Part model, mm, in its own coordinate system. A direction names the side the tool comes from. Give positions to 0.01 mm unless a question says otherwise; leave off trailing zeros. Write each loop counter-clockwise with the first axis right and the second up, starting at its lowest first coordinate (ties: lowest second). Pieces come first, ordered by that corner, then holes.
```python
from build123d import *

# Parameters (mm, degrees)
F0_W     = 5
F0_H     = 200
F1_DEPTH = 300
F2_W     = 11
F2_H     = 7
F3_DEPTH = 300
F4_R     = 3.49999
F5_W     = 15
F5_H     = 31
F6_DEPTH = 7.001
F7_R     = 2
F8_W     = 8
F8_H     = 2
F9_DEPTH = 27
F10_R    = 1.99999


# Not quite as in the source:
# - a fillet or chamfer is up to 0.001 mm smaller than in the source, because OpenCascade refuses the exact size


with BuildPart() as f1:
    # F0 (on Front) → F1 (new body)
    with BuildSketch(Plane.XZ):
        with Locations((2.5, 100)):
            Rectangle(F0_W, F0_H)
    extrude(amount=F1_DEPTH)

    # F2 (on face) → F3 (join)
    with BuildSketch(Plane.XZ.offset(300)):
        with Locations((10.5, 3.5)):
            Rectangle(F2_W, F2_H)
    extrude(amount=-F3_DEPTH)

    # F4 (radius 3.5 in the source; OpenCascade refuses exactly that, so slightly less here)
    f4_edges = [f1.edges().sort_by_distance(p)[0] for p in [
        (16, -150, 7),
        (16, -150, 0),
    ]]
    fillet(f4_edges, radius=F4_R)

    # F5 (on face) → F6 (cut, through all)
    with BuildSketch(Plane.XY.offset(7)):
        with Locations((12.5, -284.5)):
            Rectangle(F5_W, F5_H)
        with Locations((12.5, -15.5)):
            Rectangle(F5_W, F5_H)
    extrude(amount=-F6_DEPTH, mode=Mode.SUBTRACT)

    # F7
    f7_edges = [f1.edges().sort_by_distance(p)[0] for p in [
        (2.5, -300, 200),
        (2.5, 0, 200),
        (2.5, -300, 0),
        (2.5, 0, 0),
    ]]
    fillet(f7_edges, radius=F7_R)

    # F8 (on face) → F9 (cut)
    with BuildSketch(Plane.XZ.offset(269)):
        with Locations((10.5, 4.5)):
            Rectangle(F8_W, F8_H)
    extrude(amount=-F9_DEPTH, mode=Mode.SUBTRACT)

    # F10 (radius 2 in the source; OpenCascade refuses exactly that, so slightly less here)
    f10_edges = [f1.edges().sort_by_distance(p)[0] for p in [
        (14.5, -255.5, 5.5),
    ]]
    fillet(f10_edges, radius=F10_R)


solid = f1.part
```
1) Saw through at B-B, the plane z = 117.5. Write the cut outline in (x, y), then the cut area to 3 significant figures.
Answers follow:
outline: (0, -300) - (5, -300) - (5, 0) - (0, 0) - close
area: 1,500 mm2
2) Wall check: L1, parallel to X at y = -170.5, z = 145; L2, parallel to Z at x = 8.5, y = -235; L3, parallel to Z at x = 13.5, y = -268. Give the ranges that are in metal, low to high.
Answers follow:
L1: x = 0 to 5
L2: z = 0 to 7
L3: z = 0.15 to 3.5, 5.23 to 6.85
3) Pin check, flat tips, straight feed: pin 1 Ø1 at (y, z) = (-245, 168) entering from +X; pin 2 Ø2 at (x, y) = (9, -210) entering from +Z; pin 3 Ø2 at (x, z) = (9, 5) entering from -Y. Stop position of each tip, or through.
Answers follow:
pin 1: stops at x = 5
pin 2: stops at z = 7
pin 3: stops at y = -269
4) 3-axis set-ups, long thin cutter, end or side, ignore diameter. For faces 1 (the face through (10, -256, 3.5)), 2 (the face through (10, -31, 4)), 3 (the face through (10, -269, 3)), 4 (the face through (6, -152, 0)): which of +Z, -Z, +X, -X, +Y, -Y reach the whole face in a straight line?
Answers follow:
face 1: -Y
face 2: +Z, -Z, +X, +Y
face 3: +Z, -Z, +X, -Y
face 4: -Z, +X, -X, +Y, -Y
5) Saw through at C-C, the plane y = -19. Write the cut outline in (x, z), then the cut area to 3 significant figures.
Answers follow:
outline: (0, 0) - (5, 0) - (5, 200) - (0, 200) - close
area: 1,000 mm2
6) Two-plate mould, pull along X, no slides. Class faces 5 (the face through (0, -148, 99)), 6 (the face through (9, -152, 7)), 7 (the face through (9, -256, 5.5)): +X half, -X half, draft (parallel to the pull), parting line (faces both ways), or undercut.
Answers follow:
face 5: -X half
face 6: draft
face 7: undercut
